Print and shaded views of the part. All mm, measured from the part's lowest x, y and z. Round coordinates to 2 decimals unless told otherwise and drop trailing zeros. Order: outer loops, then holes, each group sorted by start corner. A loop starts at its lowest first (then second) coordinate and runs counter-clockwise, first axis right, second up. Notation, with made-up numbers: (0.25, 37) - (44.25, 37) arc R20 ccw to (44.25, 47) - close; hole circle Ø4 at (74, 39.5). An arc over 180 degrees is marked (long way). Write item = value, one per line. Start each with the question number.
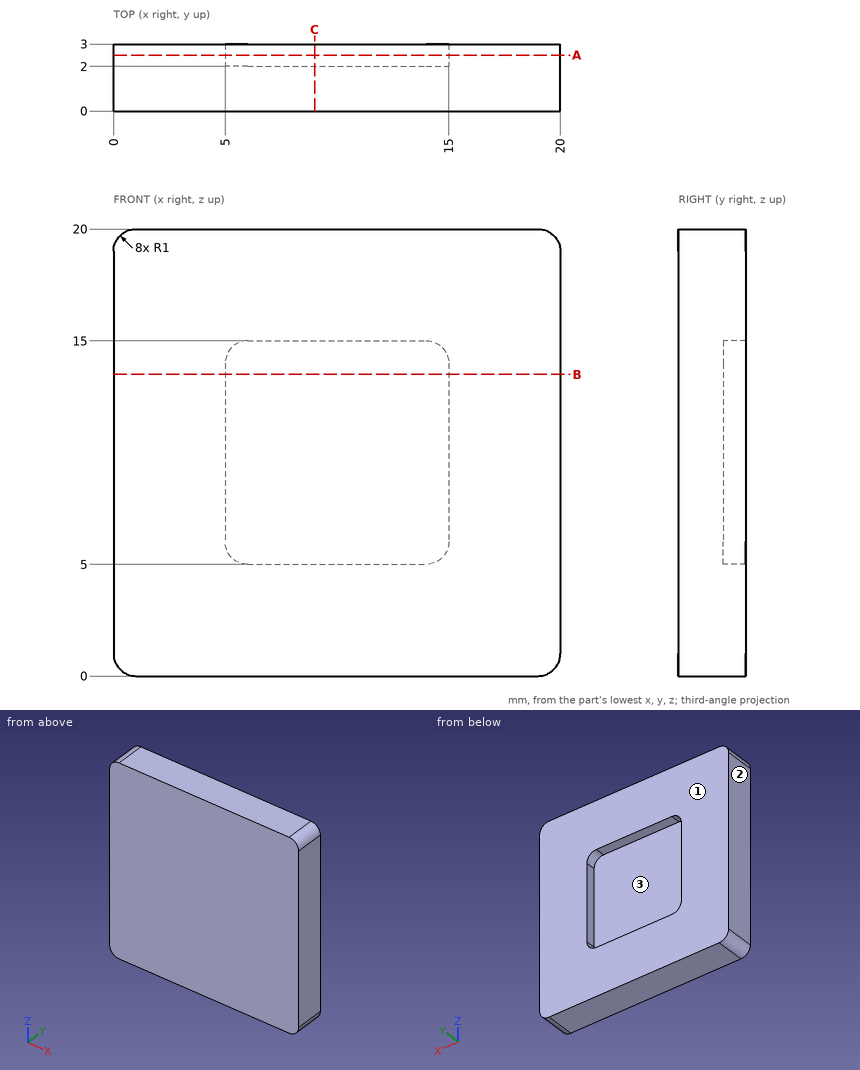
Item 1: Saw through at A-A, the plane y = 2.5. Give the cut face in (x, z).
Item 2: Mould opens along X. For the marked faces 1, 2 and 3 say: +X half, -X half, draft (parallel to the pull), parting line (faces both ways), or undercut.
Item 3: Drop a flat-ended pin along its axis: pin 1 (3 mm diameter, centred on x = 10.5, z = 7.5, fed in from +Y). Give the stop position or say it passes through.
Item 4: Saw through at C-C, the plane x = 9. Give the cut face in (y, z), then the cut area to 3 significant figures.
Item 5: Probe L1, parallel to Z at x = 10.75, y = 2.1; L2, parallel to Y at x = 8.5, z = 13.75. List the from-to ranges inside material, lowest first.
Item 6: Saw through at B-B, the plane z = 13.5. Give the cut face in (x, y).
Check sheet entries:
q1.outline = (0, 1) arc R1 ccw to (1, 0) - (19, 0) arc R1 ccw to (20, 1) - (20, 19) arc R1 ccw to (19, 20) - (1, 20) arc R1 ccw to (0, 19) - close; hole (5, 6) arc R1 ccw to (6, 5) - (14, 5) arc R1 ccw to (15, 6) - (15, 14) arc R1 ccw to (14, 15) - (6, 15) arc R1 ccw to (5, 14) - close
q2.face_1 = draft
q2.face_2 = -X half
q2.face_3 = undercut
q3.pin_1 = 2
q4.outline = (0, 0) - (3, 0) - (3, 5) - (2, 5) - (2, 15) - (3, 15) - (3, 20) - (0, 20) - close
q4.area = 50.0 mm2
q5.L1 = 0 to 5, 15 to 20
q5.L2 = 0 to 2
q6.outline = (0, 0) - (20, 0) - (20, 3) - (15, 3) - (15, 2) - (5, 2) - (5, 3) - (0, 3) - close
